from build123d import *

# Parameters (mm, degrees)
F0_W     = 50.8
F0_H     = 50.8
F1_DEPTH = 25.4
F2_W     = 38.1
F2_H     = 44.45
F3_DEPTH = 25.4
F5_DEPTH = 47.752


with BuildPart() as f1:
    # F0 (on Top) → F1 (new body)
    with BuildSketch(Plane.XY):
        Rectangle(F0_W, F0_H)
    extrude(amount=F1_DEPTH)

    # F2 (on face) → F3 (cut)
    with BuildSketch(Plane.XY.offset(25.4)):
        with Locations((0, -3.175)):
            Rectangle(F2_W, F2_H)
    extrude(amount=-F3_DEPTH, mode=Mode.SUBTRACT)

    # F4 (on face) → F5 (join)
    with BuildSketch(Plane.YZ.offset(25.4)):
        Polygon((25.4, 0), (-25.4, 25.4), (-25.4, 0), (-21.969959, 0), (-21.969959, 9.062302), align=None)
    extrude(amount=-F5_DEPTH)


solid = f1.part
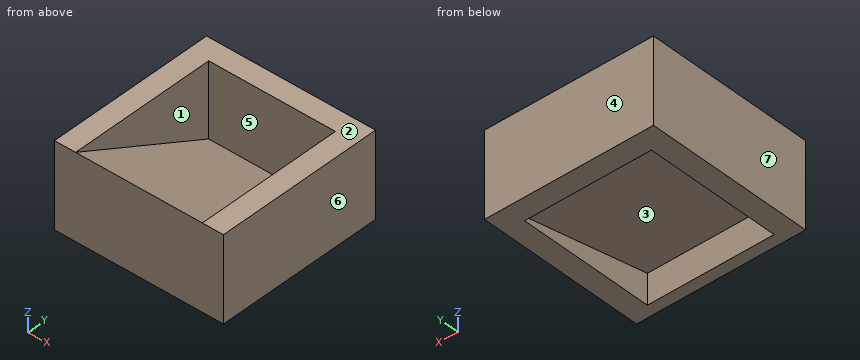
Design review of the part built by this model. Coordinates are the model's own, in mm. Face numbers are marked on the shaded views. A direction names the side the tool comes from. Coordinates: 2 decimals unless noted, no trailing zeros. Write each loop counter-clockwise with the first axis right and the second up, starting at its lowest first coordinate (ties: lowest second). Pieces come first, ordered by that corner, then holes. Notation, with made-up numbers: (86.5, -28) -> (139.5, -28) arc R32 ccw to (139.5, 9) -> close; hole circle Ø4 at (59, 21.25). An arc over 180 degrees is marked (long way). Write each question's results on one line, items separated by ' | '. Start each with the question number.
(1) Take a section at B-B on x = -11. Write out the cut boundary in (y, z) (3 decimals).
(2) Tool access review of the marked faces 1, 2 and 3: name each direction out of +Z, -Z, +X, -X, +Y, -Y from which nothing blocks a thin tool from reaching the whole face with its end or side.
(3) Clearance check with flat-ended pins moving along their axes: P1, Ø3, axis at x = 3, y = -9.5, coming from the +Z side; P2, Ø4, axis at x = -2.5, y = 12, coming from the +Z side. State where each tip first meets the part, or that it passes through.
(4) The part is to be moulded in two halves that separate along X. For the marked faces 4, 5, 6 and 7, say which applies: pulls with the +X half, pulls with the -X half, needs draft (parallel to the pull), parting line crosses it, or undercut.
(5) Take a section at A-A on z = 11.5. Write out the cut boundary in (x, y), and give its area (3 significant figures).
(6) For line 1 along X through (y, z) = (-8, 18.5); line 2 along Y through (x, z) = (-15, 1), list the stretches that pass through material, from the lowest coordinate up. Write a range as from..to.
(7) Take a section at C-C on z = 18. Write out the cut boundary in (x, y).
(8) Take a section at D-D on y = 6.5. Write out the cut boundary in (x, z), and give its area (3 significant figures).
Results found:
1) outline: (-25.4, 0) -> (-21.97, 0) -> (-21.97, 9.062) -> (19.05, 1.215) -> (19.05, 0) -> (25.4, 0) -> (25.4, 25.4) -> (19.05, 25.4) -> (19.05, 3.175) -> (-25.4, 25.4) -> close
2) face 1: +Z | face 2: +Z, +X, -X, +Y, -Y | face 3: -Z
3) P1: stops at z = 18.2 | P2: stops at z = 7.7
4) face 4: needs draft | face 5: undercut | face 6: pulls with the +X half | face 7: pulls with the -X half
5) outline: (-25.4, -25.4) -> (25.4, -25.4) -> (25.4, 25.4) -> (-25.4, 25.4) -> close; hole (-19.05, 2.4) -> (19.05, 2.4) -> (19.05, 19.05) -> (-19.05, 19.05) -> close | area: 1,950 mm2
6) line 1: x = -25.4..-19.05, 19.05..25.4 | line 2: y = -25.4..-21.97, 19.05..25.4
7) outline: (-25.4, -25.4) -> (25.4, -25.4) -> (25.4, 25.4) -> (-25.4, 25.4) -> close; hole (-19.05, -10.6) -> (19.05, -10.6) -> (19.05, 19.05) -> (-19.05, 19.05) -> close
8) outline: (-25.4, 0) -> (-19.05, 0) -> (-19.05, 3.62) -> (19.05, 3.62) -> (19.05, 0) -> (25.4, 0) -> (25.4, 25.4) -> (19.05, 25.4) -> (19.05, 9.45) -> (-19.05, 9.45) -> (-19.05, 25.4) -> (-25.4, 25.4) -> close | area: 545 mm2
